```python
from build123d import *

# Parameters (mm, degrees)
MODEL_R             = 2
MODEL_W             = 29.5
MODEL_H             = 5.5
BOSS_EXTRUDE1_DEPTH = 6


with BuildPart() as part:
    # Model → Boss-Extrude1 (new body)
    with BuildSketch(Plane.XY):
        Polygon((41.305703545, 60.317480411), (37.765395693, 64.536655013), (47.723769702, 72.891019085), (51.262213555, 68.676185328), (61.217679315, 77.034013574), (57.683186462, 81.246258129), (67.640721471, 89.601622083), (73.284512173, 91.655793907), (75.16331879, 86.492201925), (87.378490159, 90.936771689), (85.497379371, 96.105081103), (97.712550739, 100.549650868), (99.594494229, 95.383033552), (111.809665598, 99.827603316), (109.92855481, 104.995912731), (122.143726178, 109.440482495), (124.025669668, 104.27386518), (136.240841037, 108.718434944), (134.359730249, 113.886744358), (147.487562001, 118.663391555), (148.455483892, 118.663391555), (148.455483892, 113.163391555), (161.455483892, 113.163391555), (161.455483892, 118.663391555), (176.455483892, 118.663391555), (176.455483892, 113.163391555), (191.455483892, 113.163391555), (191.455483892, 118.663391555), (206.455483892, 118.663391555), (206.455483892, 113.163391555), (221.455483892, 113.163391555), (221.455483892, 118.663391555), (236.455483892, 118.663391555), (236.455483892, 113.163391555), (251.455483892, 113.163391555), (251.455483892, 118.663391555), (266.455483892, 118.663391555), (266.455483892, 113.163391555), (281.455483892, 113.163391555), (281.455483892, 118.663391555), (296.455483892, 118.663391555), (296.455483892, 113.163391555), (311.455483892, 113.163391555), (311.455483892, 100.619540915), (311.455483892, 84.936798462), (308.395932616, 69.555395508), (302.394406906, 55.066430742), (293.681542027, 42.026706955), (282.592168491, 30.937333419), (269.552444704, 22.224468541), (255.063479938, 16.22294283), (239.682076984, 13.163391555), (236.455483892, 13.163391555), (221.455483892, 13.163391555), (206.455483892, 13.163391555), (206.455483892, 7.663391555), (191.455483892, 7.663391555), (191.455483892, 13.163391555), (176.455483892, 13.163391555), (176.455483892, 7.663391555), (161.455483892, 7.663391555), (161.455483892, 13.163391555), (146.455483892, 13.163391555), (146.455483892, 7.663391555), (131.455483892, 7.663391555), (131.455483892, 13.163391555), (116.455483892, 13.163391555), (116.455483892, 7.663391555), (101.455483892, 7.663391555), (101.455483892, 13.163391555), (86.455483892, 13.163391555), (86.455483892, 7.663391555), (71.455483892, 7.663391555), (71.455483892, 13.163391555), (56.455483892, 13.163391555), (56.455483892, 7.663391555), (41.455483892, 7.663391555), (41.455483892, 13.163391555), (26.455483892, 13.163391555), (26.455483892, 7.663391555), (11.425401767, 7.663391555), (11.425401767, 35.258443505), (21.383775776, 43.612807577), (17.848443923, 47.826052014), (27.806817932, 56.180416087), (31.342353537, 51.969046503), align=None)
        with Locations((172.487562001, 88.163391555)):
            Circle(MODEL_R, mode=Mode.SUBTRACT)
        with Locations((286.455483892, 88.163391555)):
            Circle(MODEL_R, mode=Mode.SUBTRACT)
        with Locations((81.455483892, 38.163391555)):
            Circle(MODEL_R, mode=Mode.SUBTRACT)
        with Locations((172.487562001, 38.163391555)):
            Circle(MODEL_R, mode=Mode.SUBTRACT)
        with Locations((112.543046266, 78.812365745)):
            Circle(MODEL_R, mode=Mode.SUBTRACT)
        with Locations((54.155009637, 45.002140534)):
            Circle(MODEL_R, mode=Mode.SUBTRACT)
        with Locations((241.455483892, 60.413391555)):
            Rectangle(MODEL_W, MODEL_H, mode=Mode.SUBTRACT)
        Polygon((107.62898864, 62.975983599), (79.134176764, 70.61114543), (77.710672016, 65.298553385), (106.205483892, 57.663391555), align=None, mode=Mode.SUBTRACT)
    extrude(amount=BOSS_EXTRUDE1_DEPTH)


solid = part.part
```
The listing builds one solid part. Answer for the finished solid, in the listing's coordinates (mm). A direction names the side the tool comes from. Coordinates: 2 decimals unless noted, no trailing zeros. Loops run counter-clockwise (first coordinate to the right, second up) from the corner with the lowest first, then second, coordinate; pieces in that order, holes last. Notation, with made-up numbers: M -34.75,-14.5 L -12.75,-14.5 A21 cw -12.75,23.5 Z; hole C -37,-6 d3. An arc over 180 degrees is marked long. Answer as CSV lines item,"result". Start each with the question number.
(1) The part is cut by section B-B (z = 3.35). State how many separate pieces and enclosed holes the cut face has, and give its area (3 significant figures).
(2) For faces 5 (the flat face through (288.214, 36.56, 2.958)), 6 (the flat face through (49, 7.663, 3)), 7 (the flat face through (41.455, 10, 3)), 8 (the flat face through (148.455, 116, 3)), 9 (the flat face through (304, 113.163, 3)), determine the directions among +Z, -Z, +X, -X, +Y, -Y from which every point of the face is accessible in a straight line to the end or side of a thin tool.
(3) The mould has two halves that part along Y. Classify faces 1 (the flat face through (16.335, 39.377, 2.958)), 2 (the flat face through (256.205, 60, 3)), 3 (the flat face through (176.455, 116, 3)), 4 (the flat face through (199, 7.663, 3)): pulls with the +Y half, pulls with the -Y half, needs draft (parallel to the pull), parting line crosses it, or undercut.
(4) Given pin 1 (1.6 mm diameter, centred on y = 116.5, z = 4, fed in from +X); pin 2 (1 mm diameter, centred on x = 117, z = 1, fed in from -Y); pin 3 (1 mm diameter, centred on y = 51.5, z = 3, fed in from -X); pin 4 (3 mm diameter, centred on x = 81.46, y = 38.16, fed in from -Z) (3 decimals), each flat-ended and moving along its own axis, determine where each tip first touches the part or whether it passes through.
(5) Find the intervals of material crossed by L1, parallel to Y at x = 187, z = 1.75; L2, parallel to X at y = 39, z = 1.9; L3, parallel to Y at x = 92, z = 3.6, in increasing order. Write a range as [from, to].
(6) The part is cut by section A-A (x = 64.5). Give the vertices of the cut face in (y, z), and give its area (3 significant figures).
Determined:
1,separate pieces,"1"
1,enclosed holes,"8"
1,area,"25,500 mm2"
2,face 5,"+Z, -Z, +X, -Y"
2,face 6,"+Z, -Z, +X, -X, -Y"
2,face 7,"+Z, -Z, -Y"
2,face 8,"+Z, -Z, +Y"
2,face 9,"+Z, -Z, +X, +Y"
3,face 1,"undercut"
3,face 2,"undercut"
3,face 3,"needs draft"
3,face 4,"pulls with the -Y half"
4,pin 1,"x = 296.46"
4,pin 2,"y = 13.16"
4,pin 3,"x = 21.63"
4,pin 4,"through"
5,L1,"[13.16, 113.16]"
5,L2,"[15.89, 79.64], [83.27, 170.67], [174.3, 290.65]"
5,L3,"[13.16, 61.47], [67.16, 98.47]"
6,outline,"M 13.16,0 L 86.97,0 L 86.97,6 L 13.16,6 Z"
6,area,"443 mm2"
